Can you work these out from the model? Positions are in its coordinate system, mm. A direction names the side the tool comes from. Give positions to 0.01 mm unless a question says otherwise; leave off trailing zeros. Write each loop counter-clockwise with the first axis right and the second up, starting at its lowest first coordinate (ties: lowest second). Pieces come first, ordered by that corner, then holes. Notation, with made-up numbers: (4, 75.5) -> (19, 75.5) arc R21 cw to (19, 105.5) -> close; hole circle Ø5 at (-9, 19). An arc over 180 degrees is marked (long way). Answer as CSV lines item,"result". Start each with the question number.
1. I need wall thicknesses on line 1 (Y direction, x = 11, z = 118); line 2 (Z direction, x = 11.5, y = 2.75). Which ranges of each line are inside material? Lowest first, please. Write a range as [from, to].
2. If we section it at A-A on x = 3.25: Write out the boundary of the cut face in (y, z).
3. I'm going to push flat-ended pins straight in: P1, Ø5, axis at x = 9.5, y = 5.5, coming from the -Z side; P2, Ø6, axis at x = -4.5, y = 6.5, coming from the -Z side; P3, Ø3, axis at x = -10, y = -7.5, coming from the +Z side. Where does each tip first touch, or does it pass through?
4. If we section it at B-B on y = 6.75: Write out the boundary of the cut face in (x, z), plus the area to 3 significant figures.
5. On a 3-axis mill with a long thin cutter (end or side, diameter ignored), from which of +Z, -Z, +X, -X, +Y, -Y can I reach the whole of each face in a straight line? I mean faces 5 (the face through (-12.7, 0, 213)), 6 (the face through (11.112, 0, 213)). Say none if no direction works.
6. If we mould it in two halves opening along X, with no side actions, what happens to faces 1 (the face through (-11.112, 0, 213)), 2 (the face through (0, -11.112, 213)), 3 (the face through (0, -12.7, 213)), 4 (the face through (0.1, 11.3, 12.8))? For each: pulls with the +X half, pulls with the -X half, needs draft (parallel to the pull), parting line crosses it, or undercut.
7. If we section it at C-C on z = 159.5: Write out the boundary of the cut face in (x, y), plus the area to 3 significant figures.
```python
from build123d import *

# Parameters (mm, degrees)
SKETCH1_W           = 25.4
SKETCH1_H           = 25.4
SKETCH1_W_2         = 22.225
SKETCH1_H_2         = 22.225
BOSS_EXTRUDE1_DEPTH = 431.8
CUT_EXTRUDE1_DEPTH  = 433.73281595


with BuildPart() as part:
    # Sketch1 → Boss-Extrude1 (new body)
    with BuildSketch(Plane.XY):
        Rectangle(SKETCH1_W, SKETCH1_H)
        Rectangle(SKETCH1_W_2, SKETCH1_H_2, mode=Mode.SUBTRACT)
    extrude(amount=BOSS_EXTRUDE1_DEPTH)

    # Sketch2 → Cut-Extrude1 (cut, through all)
    with BuildSketch(Plane(origin=(0, 12.7, 0), x_dir=(1, 0, 0), z_dir=(0, 1, 0))):
        Polygon((12.7, 0), (12.7, -25.4), (-12.7, 0), align=None)
    cut_extrude1 = extrude(amount=-CUT_EXTRUDE1_DEPTH, mode=Mode.SUBTRACT)

    # Mirror1: Cut-Extrude1 across plane
    add(cut_extrude1.mirror(Plane.XY.offset(215.9)), mode=Mode.SUBTRACT)


solid = part.part
```
Computed values:
1,line 1,"y = [-12.7, -11.11], [11.11, 12.7]"
1,line 2,"z = [24.2, 407.6]"
2,outline,"(-12.7, 15.95) -> (-11.11, 15.95) -> (-11.11, 415.85) -> (-12.7, 415.85) -> close; (11.11, 15.95) -> (12.7, 15.95) -> (12.7, 415.85) -> (11.11, 415.85) -> close"
3,P1,"stops at z = 23.81"
3,P2,"passes through"
3,P3,"stops at z = 430.6"
4,outline,"(-12.7, 0) -> (-11.11, 1.59) -> (-11.11, 430.21) -> (-12.7, 431.8) -> close; (11.11, 23.81) -> (12.7, 25.4) -> (12.7, 406.4) -> (11.11, 407.99) -> close"
4,area,"1,290 mm2"
5,face 5,"+Z, -Z, -X, +Y, -Y"
5,face 6,"+Z, -Z"
6,face 1,"undercut"
6,face 2,"undercut"
6,face 3,"needs draft"
6,face 4,"pulls with the +X half"
7,outline,"(-12.7, -12.7) -> (12.7, -12.7) -> (12.7, 12.7) -> (-12.7, 12.7) -> close; hole (-11.11, -11.11) -> (11.11, -11.11) -> (11.11, 11.11) -> (-11.11, 11.11) -> close"
7,area,"151 mm2"
